Geometry check sheet. Reference: drawing and pictorial views, mm from the part's lowest x, y, z. A direction names the side the tool comes from. Give positions to 0.01 mm unless a question says otherwise; leave off trailing zeros. Write each loop counter-clockwise with the first axis right and the second up, starting at its lowest first coordinate (ties: lowest second). Pieces come first, ordered by that corner, then holes.
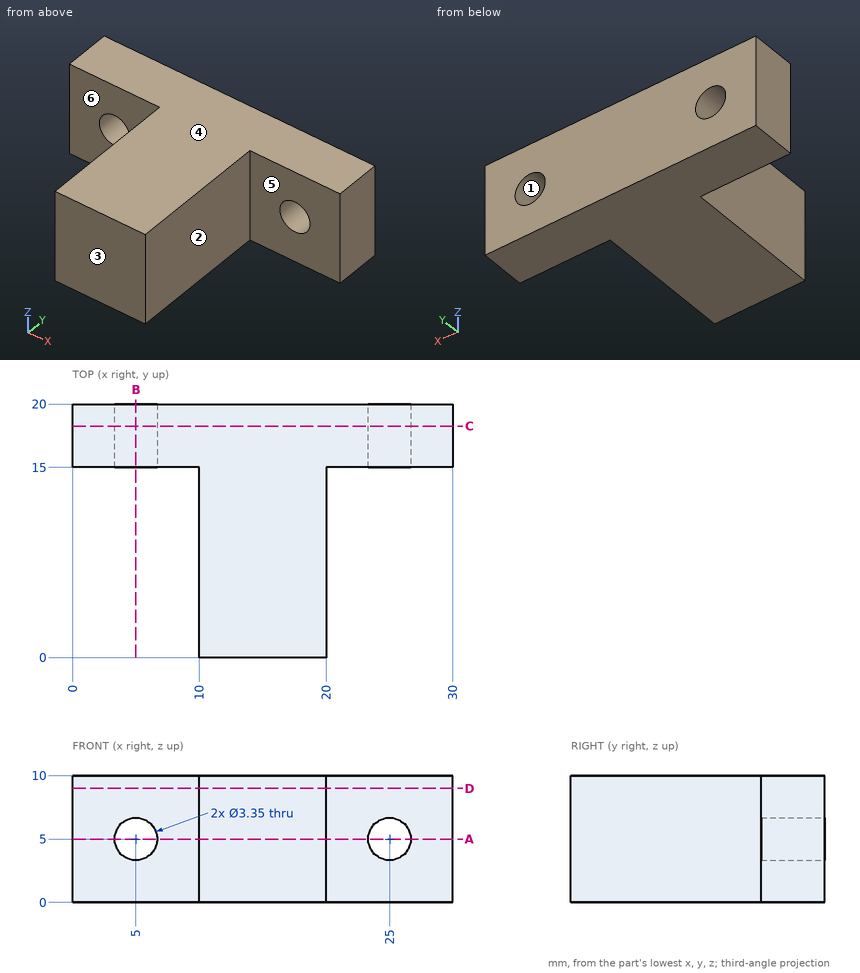
Item 1: Scan lines: line 1 along X through (y, z) = (18.95, 5) (3 decimals); line 2 along X through (y, z) = (18, 3.75) (3 decimals); line 3 along Z through (x, y) = (25, 16.15) (3 decimals). Record each from-to range of solid material in increasing order.
Answer key:
line 1: x = 0 to 3.325, 6.675 to 23.325, 26.675 to 30
line 2: x = 0 to 3.885, 6.115 to 23.885, 26.115 to 30
line 3: z = 0 to 3.325, 6.675 to 10
Item 2: Sectioned sample at C-C on y = 18.25. Record the cut outline in (x, z) (3 decimals), then the cut area to 3 significant figures.
Answer key:
outline: (0, 0) - (30, 0) - (30, 10) - (0, 10) - close; hole circle Ø3.35 at (5, 5); hole circle Ø3.35 at (25, 5)
area: 282 mm2
Item 3: Set-up check for the marked faces 4, 5 and 6: record each of +Z, -Z, +X, -X, +Y, -Y from which the full face is reachable in a straight line by a thin tool's end or side.
Answer key:
face 4: +Z, +X, -X, +Y, -Y
face 5: +Z, -Z, +X, -Y
face 6: +Z, -Z, -X, -Y
Item 4: Sectioned sample at D-D on z = 9. Record the cut outline in (x, y), then the cut area to 3 significant figures.
Answer key:
outline: (0, 15) - (10, 15) - (10, 0) - (20, 0) - (20, 15) - (30, 15) - (30, 20) - (0, 20) - close
area: 300 mm2
Item 5: Sectioned sample at A-A on z = 5. Record the cut outline in (x, y) (3 decimals).
Answer key:
outline: (0, 15) - (3.325, 15) - (3.325, 20) - (0, 20) - close; (6.675, 15) - (10, 15) - (10, 0) - (20, 0) - (20, 15) - (23.325, 15) - (23.325, 20) - (6.675, 20) - close; (26.675, 15) - (30, 15) - (30, 20) - (26.675, 20) - close
Item 6: Sectioned sample at B-B on x = 5. Record the cut outline in (y, z) (3 decimals).
Answer key:
outline: (15, 0) - (20, 0) - (20, 3.325) - (15, 3.325) - close; (15, 6.675) - (20, 6.675) - (20, 10) - (15, 10) - close
Item 7: Depth check by flat-ended pin: pin 1 (5 mm diameter, centred on y = 10, z = 3.5, fed in from +X); pin 2 (4 mm diameter, centred on y = 10.5, z = 5, fed in from -X); pin 3 (4.5 mm diameter, centred on x = 5, z = 5, fed in from -Y); pin 4 (5 mm diameter, centred on y = 15.5, z = 9, fed in from -X). Enter the tip coordinate at first touch or a pass-through.
Answer key:
pin 1: stops at x = 20
pin 2: stops at x = 10
pin 3: stops at y = 15
pin 4: stops at x = 0
Item 8: Release check for a two-part mould opening along X. For the marked faces 1, 2 and 3 record: released by +X, released by -X, zero draft, split by the parting line, or undercut.
Answer key:
face 1: undercut
face 2: released by +X
face 3: zero draft
